Part model, mm, in its own coordinate system. A direction names the side the tool comes from. Round coordinates to 2 decimals unless told otherwise and drop trailing zeros. Loops run counter-clockwise (first coordinate to the right, second up) from the corner with the lowest first, then second, coordinate; pieces in that order, holes last. Notation, with made-up numbers: M 16.5,16 L 62.5,16 A15 ccw 62.5,27 Z; hole C 49.5,-13 d1. An arc over 180 degrees is marked long. Put each result on its own line as item: value. Start each with the question number.
```python
from build123d import *

# Parameters (mm, degrees)
BOSS_EXTRUDE1_DEPTH = 200
FILLET1_R           = 3
FILLET2_R           = 3


with BuildPart() as part:
    # Sketch1 → Boss-Extrude1 (new body)
    with BuildSketch(Plane(origin=(0, 0, 0), x_dir=(1, 0, 0), z_dir=(0, 1, 0))):
        Polygon((-20, 5), (-20, 0), (0, 0), (0, 40), (-20, 40), (-20, 35), (-3, 35), (-3, 5), align=None)
        Polygon((0, 40), (0, 0), (20, 0), (20, 5), (3, 5), (3, 35), (20, 35), (20, 40), align=None)
    extrude(amount=BOSS_EXTRUDE1_DEPTH)

    # Fillet1
    fillet1_edges = [part.edges().sort_by_distance(p)[0] for p in [
        (-3, 100, -5),
        (-3, 100, -35),
        (3, 100, -35),
        (3, 100, -5),
    ]]
    fillet(fillet1_edges, radius=FILLET1_R)

    # Fillet2
    fillet2_edges = [part.edges().sort_by_distance(p)[0] for p in [
        (-20, 100, -5),
        (-20, 100, -35),
        (20, 100, -35),
        (20, 100, -5),
    ]]
    fillet(fillet2_edges, radius=FILLET2_R)


solid = part.part
```
1. Cut at A-A, the plane x = 8. Give the cut face in (y, z), and give its area (3 significant figures).
2. Which spindle directions (+Z, -Z, +X, -X, +Y, -Y) get a long thin tool onto all of the face, cutting with end or side? Do faces 1 (the flat face through (-11, 99, -5)), 2 (the flat face through (11, 99, -35)), 3 (the flat face through (1, 0, -19)). Say none if no direction does.
3. Cut at C-C, the plane z = -29. Give the cut face in (x, y).
4. Cut at B-B, the plane y = 159. Give the cut face in (x, z).
5. Mould opens along Z. For faces 4 (the flat face through (1, 200, -19)), 5 (the flat face through (-3, 99, -20)), 6 (the flat face through (0, 99, -40)) say: released by +Z, released by -Z, zero draft, split by the parting line, or undercut.
6. Drop flat-ended pins along their axis: pin 1 (1 mm diameter, centred on x = 3, y = 37.5, fed in from +Z); pin 2 (7 mm diameter, centred on y = 100.5, z = -15, fed in from -X); pin 3 (4 mm diameter, centred on y = 28.5, z = -7.5, fed in from +X); pin 4 (5 mm diameter, centred on y = 74, z = -28.5, fed in from +X). Give the stop position or say it passes through.
7. Wall check: L1, parallel to Z at x = -10, y = 86; L2, parallel to X at y = 57, z = -14; L3, parallel to Z at x = 4.5, y = 178.5. Give the ranges that are in metal, low to high.
Results list:
1. outline: M 0,-40 L 200,-40 L 200,-35 L 0,-35 Z; M 0,-5 L 200,-5 L 200,0 L 0,0 Z
1. area: 2,000 mm^2
2. face 1: -X, +Y, -Y
2. face 2: +X, +Y, -Y
2. face 3: +Z, -Z, +X, -X, -Y
3. outline: M -3,0 L 3,0 L 3,200 L -3,200 Z
4. outline: M -20,-40 L 20,-40 L 20,-38 A3 ccw 17,-35 L 6,-35 A3 cw 3,-32 L 3,-8 A3 cw 6,-5 L 17,-5 A3 ccw 20,-2 L 20,0 L -20,0 L -20,-2 A3 ccw -17,-5 L -6,-5 A3 cw -3,-8 L -3,-32 A3 cw -6,-35 L -17,-35 A3 ccw -20,-38 Z
5. face 4: zero draft
5. face 5: undercut
5. face 6: released by -Z
6. pin 1: stops at z = 0
6. pin 2: stops at x = -3
6. pin 3: stops at x = 4.34
6. pin 4: stops at x = 3
7. L1: z = -40 to -35, -5 to 0
7. L2: x = -3 to 3
7. L3: z = -40 to -34.6, -5.4 to 0
